Could you check a few things on this drawing? It's one solid part, dimensions in mm from its lowest x, y, z. A direction names the side the tool comes from. Give positions to 0.01 mm unless a question says otherwise; leave off trailing zeros. Order: outer loops, then holes, each group sorted by start corner. A loop starts at its lowest first (then second) coordinate and runs counter-clockwise, first axis right, second up. Notation, with made-up numbers: M 73,37.25 L 91,37.25 A30 cw 91,63.25 Z; hole C 65,36 d6. An arc over 180 degrees is marked long. One line per item, written item: value. Start each with the question number.
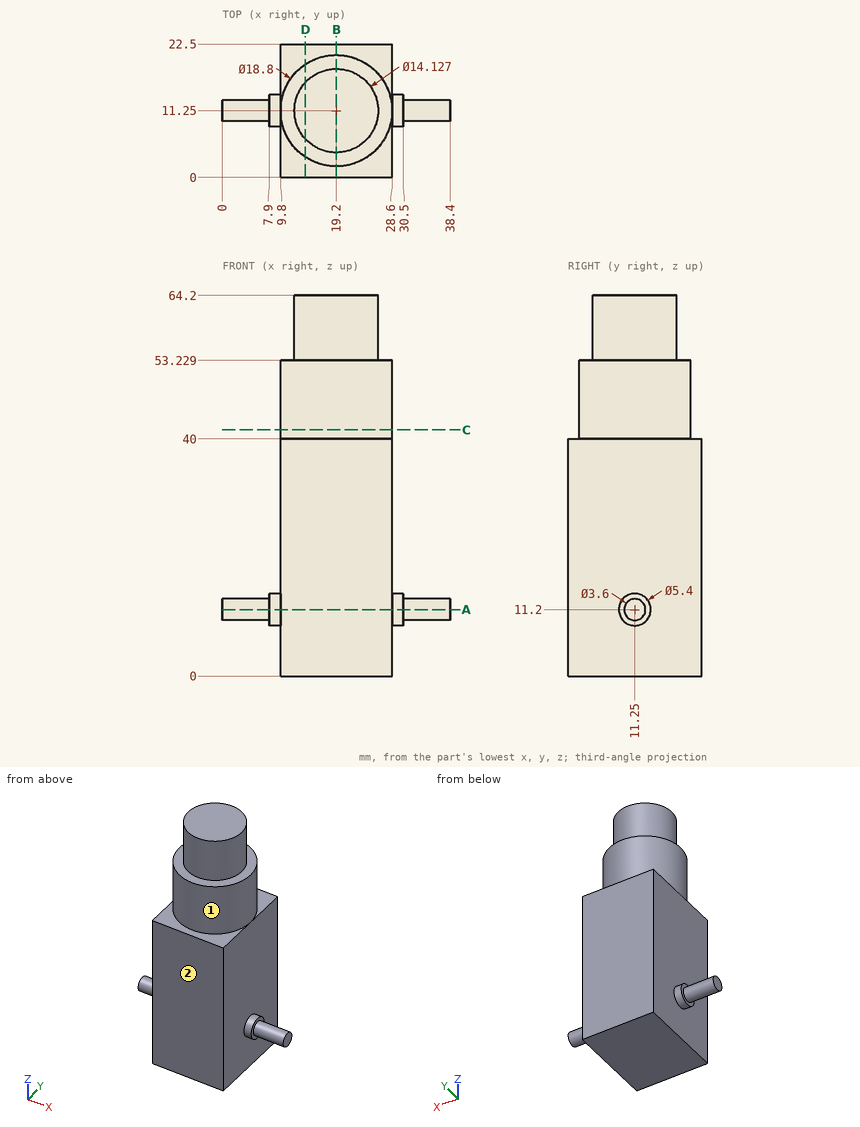
Item 1: I want a section at D-D on x = 14. Write out the boundary of the cut face in (y, z).
Item 2: Will these pins go through, and if not, where does the flat tip stop? P1, Ø1, axis at x = 15, y = 17.5, coming from the +Z side; P2, Ø5, axis at y = 2.5, z = 18, coming from the +X side; P3, Ø1, axis at y = 19.5, z = 31, coming from the -X side; P4, Ø6, axis at x = 11.5, z = 56.5, coming from the +Y side.
Item 3: For the marked faces 1 and 2, which set-ups out of +Z, -Z, +X, -X, +Y, -Y let a thin tool reach every point of the face, with its end or its side?
Item 4: I want a section at C-C on z = 41.5. Write out the boundary of the cut face in (x, y), plus the area to 3 significant figures.
Item 5: I want a section at B-B on x = 19.2. Write out the boundary of the cut face in (y, z), plus the area to 3 significant figures.
Item 6: I want a section at A-A on z = 11.2. Write out the boundary of the cut face in (x, y), plus the area to 3 significant figures.
Item 7: Please list where these lines run through material, in increasing order: probe 1 along X at (y, z) = (6.5, 24.5); probe 2 along Z at (x, y) = (24, 19.25); probe 3 along Z at (x, y) = (27.5, 16.75). Write a range as [from, to].
Answer below:
1. outline: M 0,0 L 22.5,0 L 22.5,40 L 19.08,40 L 19.08,53.23 L 16.03,53.23 L 16.03,64.2 L 6.47,64.2 L 6.47,53.23 L 3.42,53.23 L 3.42,40 L 0,40 Z
2. P1: stops at z = 64.2
2. P2: stops at x = 28.6
2. P3: stops at x = 9.8
2. P4: stops at y = 16.52
3. face 1: +Z
3. face 2: +Z, -Z, +X, -X, -Y
4. outline: C 19.2,11.25 d18.8
4. area: 278 mm²
5. outline: M 0,0 L 22.5,0 L 22.5,40 L 20.65,40 L 20.65,53.23 L 18.31,53.23 L 18.31,64.2 L 4.19,64.2 L 4.19,53.23 L 1.85,53.23 L 1.85,40 L 0,40 Z
5. area: 1,300 mm²
6. outline: M 0,9.45 L 7.9,9.45 L 7.9,8.55 L 9.8,8.55 L 9.8,0 L 28.6,0 L 28.6,8.55 L 30.5,8.55 L 30.5,9.45 L 38.4,9.45 L 38.4,13.05 L 30.5,13.05 L 30.5,13.95 L 28.6,13.95 L 28.6,22.5 L 9.8,22.5 L 9.8,13.95 L 7.9,13.95 L 7.9,13.05 L 0,13.05 Z
6. area: 500 mm²
7. probe 1: x = [9.8, 28.6]
7. probe 2: z = [0, 53.23]
7. probe 3: z = [0, 40]
